Build history of the part. All positions in model axes, mm. A direction names the side the tool comes from. Coordinates: 2 decimals unless noted, no trailing zeros. Write each loop counter-clockwise with the first axis right and the second up, starting at its lowest first coordinate (ties: lowest second). Pieces come first, ordered by that corner, then holes. Notation, with made-up numbers: (79, 49.5) -> (91, 49.5) arc R20 cw to (91, 53.5) -> close; hole circle Ø5 at (52, 55). An arc over 180 degrees is marked (long way). Write each question's results on one line, items separated by ' | '. Start each with the question number.
Q1. Tool access for faces 1 (the face through (51.32, -3.32, -0.74)), 2 (the face through (29, 9, 0)), 3 (the face through (2.03, 6.67, 7.28)): list every direction of +Z, -Z, +X, -X, +Y, -Y with a clear straight run to the whole face (end or side of a thin tool).
Q2. Drop flat-ended pins along their axis: pin 1 Ø0.7 at (x, y) = (45.5, 8.5) entering from -Z; pin 2 Ø1.5 at (x, z) = (54.5, -0.5) entering from +Y; pin 3 Ø1.1 at (x, y) = (38.5, 8.5) entering from +Z. Give the stop position or say it passes through.
Q3. Saw through at B-B on y = 9. Give the cut face in (x, z).
Q4. Saw through at D-D on x = 33. Give the cut face in (y, z).
Q5. Saw through at C-C on z = 4.5. Give the cut face in (x, y), and give its area (3 significant figures).
Q6. Two-plate mould, pull along Y, no slides. Class faces 4 (the face through (15, 10.2, 0.1)), 5 (the face through (39.84, -9.76, 2.17)), 6 (the face through (37.312, -0.576, 0.128)): released by +Y, released by -Y, zero draft, split by the parting line, or undercut.
Q7. Drill centre lines: line 1 (Y direction, x = 45, z = -0.25); line 2 (Z direction, x = 44.5, y = 0); line 3 (X direction, y = 7.75, z = 0.75). Where is each one in solid material? Low to high.
Q8. Saw through at A-A on x = 42.5. Give the cut face in (y, z), and give its area (3 significant figures).
from build123d import *

# Parameters (mm, degrees)
CUT_EXTRUDE_START     = -35
SKETCH_2_W            = 5
SKETCH_2_H            = 5
CUT_EXTRUDE_1_DEPTH   = 35
HOLE_WIZARD_M81_D     = 6.8
HOLE_WIZARD_M81_DEPTH = 25
HOLE_WIZARD_M81_TIP   = 2.042926105


with BuildPart() as part:
    # Эскиз1 → Повернуть1 (revolve)
    with BuildSketch(Plane(origin=(0, 0, 0), x_dir=(1, 0, 0), z_dir=(0, 1, 0))):
        Polygon((0, 0), (0, 9.875), (4, 9.875), (4, 12.5), (15, 12.5), (15, 10), (64, 10), (64, 0), align=None)
    revolve(axis=Axis((-1000, 0, 0), (1, 0, 0)))

    # Эскиз2 → Вырез-Вытянуть1 (cut)
    with BuildSketch(Plane(origin=(64, 0, 0), x_dir=(0, 0, -1), z_dir=(1, 0, 0)).offset(CUT_EXTRUDE_START)):
        with Locations((0, 10)):
            Rectangle(SKETCH_2_W, SKETCH_2_H)
    extrude(amount=CUT_EXTRUDE_1_DEPTH, mode=Mode.SUBTRACT)

    # Отверстие обработанное метчиком M81
    with Locations(Plane(origin=(64, 0, 0), x_dir=(0, 0, -1), z_dir=(1, 0, 0))):
        with Locations((0, 0)):
            Hole(HOLE_WIZARD_M81_D / 2, depth=HOLE_WIZARD_M81_DEPTH)
            with Locations((0, 0, -(HOLE_WIZARD_M81_DEPTH + HOLE_WIZARD_M81_TIP / 2))):  # 118° drill point
                Cone(0, HOLE_WIZARD_M81_D / 2, HOLE_WIZARD_M81_TIP, mode=Mode.SUBTRACT)


solid = part.part
Returned:
1) face 1: +X | face 2: +X, +Y | face 3: -X
2) pin 1: stops at z = -5.79 | pin 2: stops at y = 7.5 | pin 3: stops at z = 6.07
3) outline: (0, -4.06) -> (4, -4.06) -> (4, -8.67) -> (15, -8.67) -> (15, -4.36) -> (64, -4.36) -> (64, -2.5) -> (29, -2.5) -> (29, 2.5) -> (64, 2.5) -> (64, 4.36) -> (15, 4.36) -> (15, 8.67) -> (4, 8.67) -> (4, 4.06) -> (0, 4.06) -> close
4) outline: (7.5, -2.5) -> (7.5, 2.5) -> (9.68, 2.5) arc R10 ccw (long way) to (9.68, -2.5) -> close
5) outline: (0, -8.79) -> (4, -8.79) -> (4, -11.66) -> (15, -11.66) -> (15, -8.93) -> (64, -8.93) -> (64, 8.93) -> (15, 8.93) -> (15, 11.66) -> (4, 11.66) -> (4, 8.79) -> (0, 8.79) -> close | area: 1,200 mm2
6) face 4: zero draft | face 5: split by the parting line | face 6: undercut
7) line 1: y = -10 to -3.39, 3.39 to 7.5 | line 2: z = -10 to -3.4, 3.4 to 10 | line 3: x = 0 to 29
8) outline: (7.5, -2.5) -> (7.5, 2.5) -> (9.68, 2.5) arc R10 ccw (long way) to (9.68, -2.5) -> close; hole circle Ø6.8 at (0, 0) | area: 266 mm2
